The model under review builds one solid part; all positions refer to its coordinate system, in mm. A direction names the side the tool comes from. Coordinates: 2 decimals unless noted, no trailing zeros. Write each loop counter-clockwise with the first axis right and the second up, starting at its lowest first coordinate (ties: lowest second). Pieces come first, ordered by that corner, then holes. Notation, with made-up numbers: (57, -40) - (103, -40) arc R11 ccw to (103, -26) - close; hole circle Ø1 at (19.25, 75.25). An arc over 180 degrees is marked (long way). Return JSON: item names as keys, results as strings. Group by question number.
(1) For pin 1 Ø1 at (y, z) = (1, 110.5) entering from +X; pin 2 Ø1 at (x, y) = (-0.5, -5) entering from +Z; pin 3 Ø2.5 at (x, y) = (-7, -1) entering from -Z; pin 4 Ø8 at (x, z) = (6, 45) entering from +Y, all flat-tipped, find the tip position at first contact; note any pin that passes through.
(2) Tool access review of faces 1 (the face through (0, 0, 0)), 2 (the face through (0, -4, 152.4)), 3 (the face through (3, 3.175, 169)): name each direction out of +Z, -Z, +X, -X, +Y, -Y from which nothing blocks a thin tool from reaching the whole face with its end or side.
(3) Draft analysis for pull direction X (two halves, no side actions). For faces 4 (the face through (3, -3.175, 169)), 5 (the face through (1.38, 0.04, 156.36)), 6 (the face through (-2.93, 5.634, 75.133)), state which applies: released by +X, released by -X, zero draft, split by the parting line, or undercut.
(4) We need section A-A on z = 108. State the section outline as (x, y) points, then the cut area to 3 significant figures.
(5) We need section B-B on x = -11. State the section outline as (y, z) points (3 decimals).
(6) To check wall thickness, follow L1, parallel to Z at x = 0, y = -0.5; L2, parallel to X at y = -5.5, z = 58; L3, parallel to X at y = -2, z = 38.5. State the ranges of each line that lie inside material, in increasing order. Write a range as from..to.
```python
from build123d import *

# Parameters (mm, degrees)
SKETCH1_R           = 6.35
BOSS_EXTRUDE1_DEPTH = 152.4
SKETCH2_W           = 25.4
SKETCH2_H           = 6.35
BOSS_EXTRUDE2_DEPTH = 22.86
SKETCH3_R           = 6.35
CUT_EXTRUDE1_DEPTH  = 22.86


with BuildPart() as part:
    # Sketch1 → Boss-Extrude1 (new body)
    with BuildSketch(Plane.XY):
        with Locations(Location((0, 0, 0), (0, 0, 180))):
            Circle(SKETCH1_R)
    extrude(amount=BOSS_EXTRUDE1_DEPTH)

    # Sketch2 → Boss-Extrude2 (add)
    with BuildSketch(Plane.XY.offset(152.4)):
        Rectangle(SKETCH2_W, SKETCH2_H)
    extrude(amount=BOSS_EXTRUDE2_DEPTH)

    # Sketch3 → Cut-Extrude1 (cut)
    with BuildSketch(Plane(origin=(0, 3.175, 0), x_dir=(1, 0, 0), z_dir=(0, 1, 0))):
        with Locations(Location((0, -162.56, 0), (0, 0, 180))):
            Circle(SKETCH3_R)
        with BuildLine():
            ThreePointArc((12.7, -162.56), (8.980256121, -171.540256121), (0, -175.26))
            Line((0, -175.26), (12.7, -175.26))
            Line((12.7, -175.26), (12.7, -162.56))
        make_face()
        with BuildLine():
            Line((-12.7, -175.26), (0, -175.26))
            ThreePointArc((0, -175.26), (-8.980256121, -171.540256121), (-12.7, -162.56))
            Line((-12.7, -162.56), (-12.7, -175.26))
        make_face()
        with BuildLine():
            ThreePointArc((7.62, -152.4), (11.359225326, -156.880387337), (12.7, -162.56))
            Line((12.7, -162.56), (12.7, -152.4))
            Line((12.7, -152.4), (7.62, -152.4))
        make_face()
        with BuildLine():
            Line((-12.7, -152.4), (-12.7, -162.56))
            ThreePointArc((-12.7, -162.56), (-11.359225326, -156.880387337), (-7.62, -152.4))
            Line((-7.62, -152.4), (-12.7, -152.4))
        make_face()
    extrude(amount=-CUT_EXTRUDE1_DEPTH, mode=Mode.SUBTRACT)


solid = part.part
```
Ans:
{
 "1": {"pin 1": "x = 6.33", "pin 2": "z = 152.4", "pin 3": "z = 0", "pin 4": "y = 6.03"},
 "2": {"face 1": "-Z, +X, -X, +Y, -Y", "face 2": "+Z, +X, -X, -Y", "face 3": "+Z, +X, -X, +Y"},
 "3": {"face 4": "zero draft", "face 5": "undercut", "face 6": "split by the parting line"},
 "4": {"outline": "circle Ø12.7 at (0, 0)", "area": "127 mm²"},
 "5": {"outline": "(-3.175, 156.213) - (3.175, 156.213) - (3.175, 168.907) - (-3.175, 168.907) - close"},
 "6": {"L1": "0..156.21, 168.91..175.26", "L2": "-3.17..3.17", "L3": "-6.03..6.03"}
}
